```python
from build123d import *

# Parameters (mm, degrees)
F1_DEPTH = 304.8
F5_R     = 25.4
F5_R_2   = 23.114
F8_DEPTH = 2.286


# Not quite as in the source:
# - a pattern or mirror of a feature is missing from the dataset's text; its kind, count and spacing are read off the source's solid


with BuildPart() as f1:
    # F0 (on Front) → F1 (new body)
    with BuildSketch(Plane.XZ):
        with BuildLine():
            ThreePointArc((-36.8149627644, 6.858), (-36.8149627644, 2.286), (-32.8554946183, 0))
            Line((-32.8554946183, 0), (32.8554946183, 0))
            ThreePointArc((32.8554946183, 0), (36.8149627644, 2.286), (36.8149627644, 6.858))
            Line((36.8149627644, 6.858), (26.1097340731, 25.4))
            Line((26.1097340731, 25.4), (24.13, 24.257))
            Line((24.13, 24.257), (34.8352286913, 5.715))
            ThreePointArc((34.8352286913, 5.715), (34.8352286913, 3.429), (32.8554946183, 2.286))
            Line((32.8554946183, 2.286), (-32.8554946183, 2.286))
            ThreePointArc((-32.8554946183, 2.286), (-34.8352286913, 3.429), (-34.8352286913, 5.715))
            Line((-34.8352286913, 5.715), (-24.13, 24.257))
            Line((-24.13, 24.257), (-26.1097340731, 25.4))
            Line((-26.1097340731, 25.4), (-36.8149627644, 6.858))
        make_face()
    extrude(amount=F1_DEPTH)

    # F6: sweep along a path in F3
    with BuildLine(Plane.YZ) as f6_path:
        Line((-152.4, 0), (-152.4, -374.65))
        ThreePointArc((-152.4, -374.65), (-131.9414086659, -424.0414086659), (-82.55, -444.5))
    # F5 (on plane+point) → F6 (sweep)
    with BuildSketch(Plane.XZ.offset(82.55)):
        with Locations((0, -444.5)):
            Circle(F5_R)
        with Locations((0, -444.5)):
            Circle(F5_R_2, mode=Mode.SUBTRACT)
    sweep(path=f6_path.line)

    # F7 (on face) → F8 (cut, through all)
    with BuildSketch(Plane(origin=(30.5808231829, 0, 17.6558464967), x_dir=(0, 1, 0), z_dir=(0.8660254038, 0, 0.5))):
        with BuildLine():
            Line((-254, 2.5921782196), (-279.4, 2.5921782196))
            ThreePointArc((-279.4, 2.5921782196), (-282.575, -0.5828217804), (-279.4, -3.7578217804))
            Line((-279.4, -3.7578217804), (-254, -3.7578217804))
            ThreePointArc((-254, -3.7578217804), (-250.825, -0.5828217804), (-254, 2.5921782196))
        make_face()
        with BuildLine():
            Line((-139.7, 2.5921782196), (-165.1, 2.5921782196))
            ThreePointArc((-165.1, 2.5921782196), (-168.275, -0.5828217804), (-165.1, -3.7578217804))
            Line((-165.1, -3.7578217804), (-139.7, -3.7578217804))
            ThreePointArc((-139.7, -3.7578217804), (-136.525, -0.5828217804), (-139.7, 2.5921782196))
        make_face()
        with BuildLine():
            ThreePointArc((-25.4, -3.7578217804), (-22.225, -0.5828217804), (-25.4, 2.5921782196))
            Line((-25.4, 2.5921782196), (-50.8, 2.5921782196))
            ThreePointArc((-50.8, 2.5921782196), (-53.975, -0.5828217804), (-50.8, -3.7578217804))
            Line((-50.8, -3.7578217804), (-25.4, -3.7578217804))
        make_face()
    f8 = extrude(amount=-F8_DEPTH, mode=Mode.SUBTRACT)

    # F8_copies: F8 across plane
    add(f8.mirror(Plane(origin=(0, 0, 0), x_dir=(0, 0, -1), z_dir=(-1, 0, 0))), mode=Mode.SUBTRACT)


solid = f1.part
```
For this review, take the finished solid that the model builds, in its own axes (mm). A direction names the side the tool comes from. Give positions to 0.01 mm unless a question says otherwise; leave off trailing zeros. Write each loop counter-clockwise with the first axis right and the second up, starting at its lowest first coordinate (ties: lowest second). Pieces come first, ordered by that corner, then holes. Notation, with made-up numbers: M 0,5.5 L 44,5.5 A33 cw 44,40.5 Z; hole C -20,-28 d6. An arc over 180 degrees is marked long. Answer as a JSON object with one key per item and string values. Group by question number.
Item 1: Consider section D-D on x = 0. Write out the cut boundary in (y, z).
Item 2: For probe 1 along X at (y, z) = (-152, -268); probe 2 along Y at (x, z) = (0, -262.5); probe 3 along Z at (x, y) = (-15, -139.5), list the stretches that pass through material, from the lowest coordinate up. Write a range as [from, to].
Item 3: Consider section A-A on y = -152.4. Count the separate pieces of the cut face and the enclosed holes in it, plus the area to 3 significant figures.
Item 4: Tool access review of faces 4 (the flat face through (-21, -82.55, -456)), 5 (the flat face through (0, -152, 0)), 6 (the flat face through (0, -150, 2.286)): name each direction out of +Z, -Z, +X, -X, +Y, -Y from which nothing blocks a thin tool from reaching the whole face with its end or side.
Item 5: For pin 1 Ø1.5 at (x, z) = (7.5, -273.5) entering from +Y; pin 2 Ø6 at (y, z) = (-183, -81.5) entering from -X; pin 3 Ø14 at (x, y) = (4, -155.5) entering from -Z; pin 4 Ø10 at (x, y) = (10, -100.5) entering from -Z, all flat-tipped, find the tip position at first contact; note any pin that passes through.
Item 6: Consider section B-B on y = -186. Write out the cut boundary in (x, z) (1 decimal), plus the area to 3 significant figures.
Item 7: Consider section C-C on z = -247. Write out the cut boundary in (x, y), plus the area to 3 significant figures.
Item 8: Draft analysis for pull direction X (two halves, no side actions). For faces 1 (the flat face through (32.727, -150.266, 13.939)), 2 (the flat face through (3, 0, 1)), 3 (the flat face through (-30.747, -150.266, 12.796)), state which applies: +X half, -X half, draft (parallel to the pull), parting line (faces both ways), or undercut.
Check result:
{
 "1": {"outline": "M -304.8,0 L -177.8,0 L -177.8,-374.65 A95.25 ccw -82.55,-469.9 L -82.55,-467.61 A92.96 cw -175.51,-374.65 L -175.51,0 L -129.29,0 L -129.29,-374.65 A46.74 ccw -82.55,-421.39 L -82.55,-419.1 A44.45 cw -127,-374.65 L -127,0 L 0,0 L 0,2.29 L -304.8,2.29 Z"},
 "2": {"probe 1": "x = [-25.4, -23.11], [23.11, 25.4]", "probe 2": "y = [-177.8, -175.51], [-129.29, -127]", "probe 3": "z = [-444.79, -441], [0, 2.29]"},
 "3": {"separate pieces": "3", "enclosed holes": "1", "area": "2,350 mm^2"},
 "4": {"face 4": "-Z, +X, -X, +Y", "face 5": "none", "face 6": "+Y, -Y"},
 "5": {"pin 1": "stops at y = -127.91", "pin 2": "passes through", "pin 3": "stops at z = -443.06", "pin 4": "stops at z = -467.99"},
 "6": {"outline": "M -36.8,6.9 A4.6 ccw -32.9,0 L 32.9,0 A4.6 ccw 36.8,6.9 L 26.1,25.4 L 24.1,24.3 L 34.8,5.7 A2.3 cw 32.9,2.3 L -32.9,2.3 A2.3 cw -34.8,5.7 L -24.1,24.3 L -26.1,25.4 Z", "area": "281 mm^2"},
 "7": {"outline": "C 0,-152.4 d50.8; hole C 0,-152.4 d46.23", "area": "348 mm^2"},
 "8": {"face 1": "+X half", "face 2": "draft", "face 3": "undercut"}
}
